Geometry: final body of the model. Coordinates: model frame, mm. Face numbers are marked on the shaded views. A direction names the side the tool comes from. Give positions to 0.01 mm unless a question says otherwise; leave off trailing zeros. Order: outer loops, then holes, each group sorted by start corner. A loop starts at its lowest first (then second) coordinate and runs counter-clockwise, first axis right, second up. Notation, with made-up numbers: (28.5, 81.25) -> (79.5, 81.25) arc R26 ccw to (79.5, 117.25) -> close; hole circle Ø5 at (-39, 85). An arc over 180 degrees is marked (long way). Write item = value, one per line.
```python
from build123d import *

# Parameters (mm, degrees)
F1_DEPTH = 30
F3_W     = 1.5
F3_H     = 8
F4_DEPTH = 8
F5_R     = 2.5
F6_DEPTH = 13
F7_R     = 3.99999


# Not quite as in the source:
# - a fillet or chamfer is up to 0.001 mm smaller than in the source, because OpenCascade refuses the exact size


with BuildPart() as f1:
    # F0 (on Front) → F1 (new body)
    with BuildSketch(Plane.XZ):
        Polygon((-14, 0), (0, 0), (0, 5), (-0.5, 5), (-2, 5), (-12, 5), (-13.5, 5), (-14, 5), align=None)
    extrude(amount=F1_DEPTH)

    # F3 (on offset) → F4 (join)
    with BuildSketch(Plane.XZ.offset(25)):
        with Locations((-12.75, 9)):
            Rectangle(F3_W, F3_H)
        with Locations((-1.25, 9)):
            Rectangle(F3_W, F3_H)
    extrude(amount=-F4_DEPTH)

    # F5 (on face) → F6 (join, through all)
    with BuildSketch(Plane.YZ.offset(-0.5)):
        with Locations((-21, 9)):
            Circle(F5_R)
    extrude(amount=-F6_DEPTH)

    # F7 (radius 4 in the source; OpenCascade refuses exactly that, so slightly less here)
    f7_edges = [f1.edges().sort_by_distance(p)[0] for p in [
        (-1.25, -17, 13),
        (-1.25, -25, 13),
        (-12.75, -17, 13),
        (-12.75, -25, 13),
    ]]
    fillet(f7_edges, radius=F7_R)


solid = f1.part
```
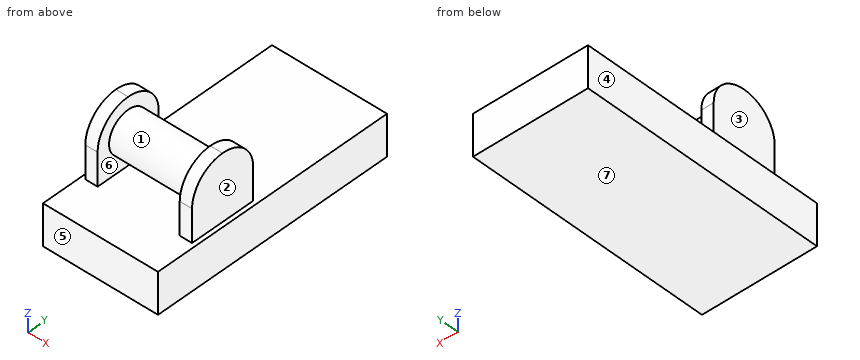
1) Section query C-C (y = -16). Output: boundary loops of the cut face in (x, z).
Check sheet entries:
outline = (-14, 0) -> (0, 0) -> (0, 5) -> (-14, 5) -> close
2) Mould query, pull axis Z, two halves, no side actions, for the marked faces 5, 6 and 7. Classes: +Z half, -Z half, draft (parallel to the pull), parting line (faces both ways), or undercut.
Check sheet entries:
face_5 = draft
face_6 = undercut
face_7 = -Z half
3) First-contact query: P1, Ø1.2, axis at x = -1.5, z = 6.5, coming from the -Y side; P2, Ø5, axis at y = -12.5, z = 9, coming from the -X side; P3, Ø6, axis at y = -23.5, z = 8.5, coming from the +X side; P4, Ø1, axis at x = -7.5, y = -19, coming from the +Z side. Flat tips, straight axial feed; report the tip coordinate or a pass-through.
Check sheet entries:
P1 = -25
P2 = through
P3 = -0.5
P4 = 11
4) Section query A-A (x = -9). Output: boundary loops of the cut face in (y, z).
Check sheet entries:
outline = (-30, 0) -> (0, 0) -> (0, 5) -> (-30, 5) -> close; circle Ø5 at (-21, 9)
5) Line query: line 1 (X direction, y = -20.75, z = 12.25); line 2 (Z direction, x = -4.5, y = -4); line 3 (Y direction, x = -1, z = 9.25). Output: solid intervals per line, ascending. Write a range as from..to.
Check sheet entries:
line_1 = -13.5..-12, -2..-0.5
line_2 = 0..5
line_3 = -24.99..-17.01
6) Reachability of the marked faces 1, 2, 3 and 4 from +Z, -Z, +X, -X, +Y, -Y: full face, straight path, thin tool, end or side. Return the list, or none.
Check sheet entries:
face_1 = none
face_2 = +Z, +X, +Y, -Y
face_3 = +Z, -X, +Y, -Y
face_4 = +Z, -Z, -X, +Y, -Y
